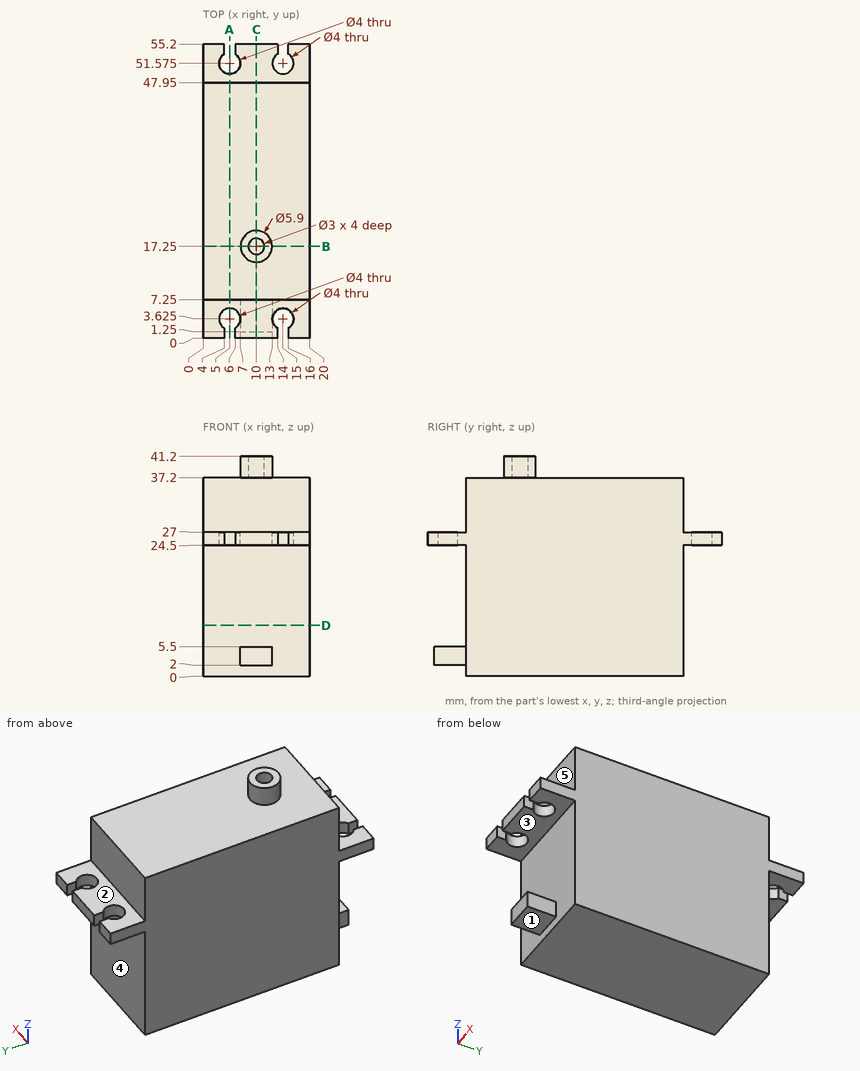
Geometry: see drawing. Coordinates: mm, zero at the bounding-box minimum. A direction names the side the tool comes from. Coordinates: 2 decimals unless noted, no trailing zeros. Loops run counter-clockwise (first coordinate to the right, second up) from the corner with the lowest first, then second, coordinate; pieces in that order, holes last.
Q1. Cut plane A-A (x = 5). Output: boundary loops of the cut face in (y, z) (3 decimals).
Q2. Cut plane B-B (y = 17.25). Output: boundary loops of the cut face in (x, z), then the cut area to 3 significant figures.
Q3. Material intervals for line 1 (Y direction, x = 8.5, z = 11); line 2 (Z direction, x = 6.75, y = 47); line 3 (Y direction, x = 5, z = 25.8) (3 decimals), sorted ascending.
Q4. Set-up query: the marked faces 1, 2, 3, 4 and 5. Return all of +Z, -Z, +X, -X, +Y, -Y with unobstructed straight access to the full face (end or side cutting, diameter ignored); none if empty.
Q5. Cut plane D-D (z = 9.5). Output: boundary loops of the cut face in (x, y).
Q6. Contact query for flat-ended pins moving along their axis: pin 1 (4.5 mm diameter, centred on x = 5, y = 3.625, fed in from +Z); pin 2 (1.5 mm diameter, centred on x = 10.5, y = 16, fed in from +Z); pin 3 (6 mm diameter, centred on x = 12.5, y = 33, fed in from +Z); pin 4 (2 mm diameter, centred on x = 9, z = 21, fed in from +Y). Output: stop coordinate, or through.
Q7. Cut plane C-C (x = 10). Output: boundary loops of the cut face in (y, z), then the cut area to 3 significant figures.
Working result:
1. outline: (5.625, 24.5) - (7.25, 24.5) - (7.25, 0) - (47.95, 0) - (47.95, 24.5) - (49.575, 24.5) - (49.575, 27) - (47.95, 27) - (47.95, 37.2) - (7.25, 37.2) - (7.25, 27) - (5.625, 27) - close
2. outline: (0, 0) - (20, 0) - (20, 37.2) - (12.95, 37.2) - (12.95, 41.2) - (11.5, 41.2) - (11.5, 37.2) - (8.5, 37.2) - (8.5, 41.2) - (7.05, 41.2) - (7.05, 37.2) - (0, 37.2) - close
2. area: 756 mm2
3. line 1: y = 7.25 to 47.95
3. line 2: z = 0 to 37.2
3. line 3: y = 5.625 to 49.575
4. face 1: -Z, +X, -X, -Y
4. face 2: +Z, +X, -X, +Y
4. face 3: +X, -X, -Y
4. face 4: -Z, +X, -X, +Y
4. face 5: +Z, +X, -X, -Y
5. outline: (0, 7.25) - (20, 7.25) - (20, 47.95) - (0, 47.95) - close
6. pin 1: stops at z = 27
6. pin 2: stops at z = 41.2
6. pin 3: stops at z = 37.2
6. pin 4: stops at y = 47.95
7. outline: (0, 24.5) - (7.25, 24.5) - (7.25, 5.5) - (1.25, 5.5) - (1.25, 2) - (7.25, 2) - (7.25, 0) - (47.95, 0) - (47.95, 24.5) - (55.2, 24.5) - (55.2, 27) - (47.95, 27) - (47.95, 37.2) - (20.2, 37.2) - (20.2, 41.2) - (18.75, 41.2) - (18.75, 37.2) - (15.75, 37.2) - (15.75, 41.2) - (14.3, 41.2) - (14.3, 37.2) - (7.25, 37.2) - (7.25, 27) - (0, 27) - close
7. area: 1,580 mm2
